Input: part model. Units: mm. Frame: model coordinates. A direction names the side the tool comes from. Give positions to 0.01 mm unless a question says otherwise; leave off trailing zeros. Order: outer loops, then holes, each group sorted by start corner. A loop starts at its lowest first (then second) coordinate and runs counter-clockwise, first axis right, second up. Notation, with made-up numbers: M 38.25,8.25 L 80.25,8.25 A24 cw 80.25,33.25 Z; hole C -14.75,-4 d2. An arc over 180 degrees is marked long. Use a Markdown table: item, result.
from build123d import *

# Parameters (mm, degrees)
PAD_DEPTH       = 8
CHAMFER_SIZE    = 2
SKETCH002_R     = 2.6
POCKET_DEPTH    = 1.6
SKETCH003_R     = 1.7
POCKET001_DEPTH = 8
POCKET002_DEPTH = 1.175


with BuildPart() as part:
    # Sketch → Revolution (revolve)
    with BuildSketch(Plane.XY):
        with BuildLine():
            Line((0, -2), (28.3, -2))
            Line((28.3, -2), (33.3, 3))
            Line((33.3, 3), (36.5, 3))
            Line((36.5, 3), (36.5, 2.12132))
            Line((36.5, 2.12132), (35.43934, 1.06066))
            ThreePointArc((35.43934, 1.06066), (35, 0), (35.43934, -1.06066))
            Line((35.43934, -1.06066), (36.5, -2.12132))
            Line((36.5, -2.12132), (36.5, -3))
            Line((36.5, -3), (35.1, -4.4))
            Line((35.1, -4.4), (0, -4.4))
            Line((0, -4.4), (0, -2))
        make_face()
    revolve(axis=Axis((0, 0, 0), (0, 1, 0)))

    # Sketch001 (on Face1 of Revolution) → Pad (new body)
    with BuildSketch(Plane(origin=(0, -2, 0), x_dir=(-1, 0, 0), z_dir=(0, 1, 0))):
        with BuildLine():
            Line((4.5, 8.125), (-4.5, 8.125))
            Line((-4.5, 8.125), (-6.893963, 4.058728))
            ThreePointArc((-6.893963, 4.058728), (0, -8), (6.893963, 4.058728))
            Line((6.893963, 4.058728), (4.5, 8.125))
        make_face()
        with BuildLine():
            Line((-2.04939, 1.6), (2.04939, 1.6))
            ThreePointArc((2.04939, -1.6), (2.6, 0), (2.04939, 1.6))
            Line((-2.04939, -1.6), (2.04939, -1.6))
            ThreePointArc((-2.04939, 1.6), (-2.6, 0), (-2.04939, -1.6))
        make_face(mode=Mode.SUBTRACT)
    extrude(amount=PAD_DEPTH)

    # Chamfer
    chamfer_edges = [part.edges().sort_by_distance(p)[0] for p in [
        (0, -2, -8),
    ]]
    chamfer(chamfer_edges, length=CHAMFER_SIZE)

    # Sketch002 (on Face8 of Chamfer) → Pocket (cut)
    with BuildSketch(Plane(origin=(0, 6, 0), x_dir=(-1, 0, 0), z_dir=(0, 1, 0))):
        Circle(SKETCH002_R)
    extrude(amount=-POCKET_DEPTH, mode=Mode.SUBTRACT)

    # Sketch003 (on Face8 of Pocket) → Pocket001 (cut)
    with BuildSketch(Plane.XY.offset(8.125)):
        with Locations((0, 2)):
            Circle(SKETCH003_R)
    extrude(amount=-POCKET001_DEPTH, mode=Mode.SUBTRACT)

    # Sketch004 (on Face9 of Pocket001) → Pocket002 (cut, symmetric)
    with BuildSketch(Plane.XY.offset(5.3875)):
        Polygon((-2.8, 0.016581), (-2.8, 6.016581), (2.8, 6.016581), (2.8, 0.016581), (0, -1.6), align=None)
    extrude(amount=POCKET002_DEPTH, both=True, mode=Mode.SUBTRACT)


solid = part.part
1) Mould query, pull axis Z, two halves, no side actions, for faces 1 (the face through (-7.912, 2.555, 35.632)), 2 (the face through (-30, 3, 16)), 3 (the face through (0.2, -0.3, -8.3)). Classes: released by +Z, released by -Z, zero draft, split by the parting line, or undercut.
Response values:
| item | result |
|---|---|
| face 1 | split by the parting line |
| face 2 | zero draft |
| face 3 | undercut |
2) First-contact query: pin 1 Ø4.5 at (x, y) = (0, 2) entering from -Z; pin 2 Ø2.5 at (y, z) = (4.5, 6) entering from -X; pin 3 Ø1.2 at (x, y) = (-0.5, 0) entering from +Z. Flat tips, straight axial feed; report the tip coordinate or a pass-through.
Response values:
| item | result |
|---|---|
| pin 1 | stops at z = -36.5 |
| pin 2 | stops at x = -6.49 |
| pin 3 | stops at z = 35.12 |
3) Cut plane A-A on z = 0. Return loops of the section in (x, y), and give its area (3 significant figures).
Response values:
| item | result |
|---|---|
| outline | M -36.5,-3 L -35.1,-4.4 L 35.1,-4.4 L 36.5,-3 L 36.5,-2.12 L 35.44,-1.06 A1.5 cw 35.44,1.06 L 36.5,2.12 L 36.5,3 L 33.3,3 L 28.3,-2 L 10,-2 L 8,0 L 8,6 L 2.6,6 L 2.6,-2 L -2.6,-2 L -2.6,6 L -8,6 L -8,0 L -10,-2 L -28.3,-2 L -33.3,3 L -36.5,3 L -36.5,2.12 L -35.44,1.06 A1.5 cw -35.44,-1.06 L -36.5,-2.12 Z |
| area | 313 mm² |
4) Material intervals for line 1 (Y direction, x = 0, z = 2); line 2 (Y direction, x = 0, z = 3.6); line 3 (Z direction, x = 26, y = 0), sorted ascending. Write a range as from..to.
Response values:
| item | result |
|---|---|
| line 1 | y = -4.4..0.3, 3.7..4.4 |
| line 2 | y = -4.4..0.3, 3.7..6 |
| line 3 | z = -23.43..-15.56, 15.56..23.43 |
5) Reachability of faces 4 (the face through (0, -4.4, 0)), 5 (the face through (0, 1, -1.6)), 6 (the face through (-1.25, 3.15, 2.92)) from +Z, -Z, +X, -X, +Y, -Y: full face, straight path, thin tool, end or side. Return the list, or none.
Response values:
| item | result |
|---|---|
| face 4 | +Z, -Z, +X, -X, -Y |
| face 5 | +Y |
| face 6 | none |
